The listing builds one solid part. Answer for the finished solid, in the listing's coordinates (mm). Round coordinates to 2 decimals unless told otherwise and drop trailing zeros. Write each loop counter-clockwise with the first axis right and the second up, starting at its lowest first coordinate (ties: lowest second). Pieces come first, ordered by that corner, then holes.
Item 1: Find section B-B on y = 1.8. Give the vertices of the cut face in (x, z).
Item 2: Find section A-A on z = 25. Give the vertices of the cut face in (x, y), then the cut area to 3 significant figures.
Item 3: This flat-tipped pin is pushed along its axis until it touches: pin 1 (3.5 mm diameter, centred on x = 25.83, z = -25.83, fed in from -Y). Where does it stop, or does it pass through?
Item 4: Find the intervals of material crossed by probe 1 along Z at (x, y) = (-25, 3.4); probe 2 along Z at (x, y) = (-28, 2.3); probe 3 along X at (y, z) = (3.1, 28.5), in increasing order.
Autodesk Inventor part; units mm, degrees
ref_plane "YZ Plane" through (0, 0, 0) normal (1, 0, 0) x (0, 1, 0)
ref_plane "XZ Plane" through (0, 0, 0) normal (0, 1, 0) x (-1, 0, 0)
ref_plane "XY Plane" through (0, 0, 0) normal (0, 0, 1) x (1, 0, 0)
sketch "Sketch1" plane through (0, 0, 0) normal (0, 1, 0) x (-1, 0, 0)
  line L0 (25.8285, 25.8285) -> (-25.8285, 25.8285) construction
  line L1 (-25.8285, 25.8285) -> (-25.8285, -25.8285) construction
  line L2 (-25.8285, -25.8285) -> (25.8285, -25.8285) construction
  line L3 (25.8285, -25.8285) -> (25.8285, 25.8285) construction
  line L4 (25.8285, 25.8285) -> (-25.8285, -25.8285) construction
  line L5 (-25.8285, 25.8285) -> (25.8285, -25.8285) construction
  line L6 (31, 26.3139) -> (31, -26.3139)
  line L7 (25.8285, -25.8285) -> (28.6569, -28.6569) construction
  line L8 (28.6569, -28.6569) -> (31, -26.3139)
  line L9 (0, 0) -> (14.4135, 0) construction
  line L10 (25.8285, 25.8285) -> (28.6569, 28.6569) construction
  line L11 (28.6569, 28.6569) -> (31, 26.3139)
  line L12 (-26.3139, 31) -> (26.3139, 31)
  line L13 (28.6569, 28.6569) -> (26.3139, 31)
  line L14 (-28.6569, 28.6569) -> (-26.3139, 31)
  line L15 (-31, -26.3139) -> (-31, 26.3139)
  line L16 (-28.6569, 28.6569) -> (-31, 26.3139)
  line L17 (-28.6569, -28.6569) -> (-31, -26.3139)
  line L18 (26.3139, -31) -> (-26.3139, -31)
  line L19 (-28.6569, -28.6569) -> (-26.3139, -31)
  line L20 (28.6569, -28.6569) -> (26.3139, -31)
  dimension "d0" = 51.657
  dimension "d1" = 51.657
  dimension "d4" = 31
  dimension "d5" = 4
  dimension "d8" = 360
extrude "Extrusion1" add sketch "Sketch1" along normal blind 4
hole "Hole1" at (-25.8285, 0, 25.8285) at (-25.8285, 0, -25.8285) at (25.8285, 0, 25.8285) at (25.8285, 0, -25.8285) direction (0, 1, 0) diameter 4.2 end through all
properties part number "top"
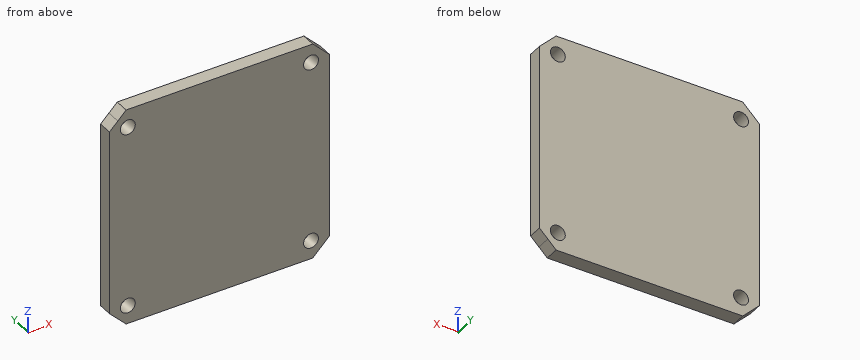
Check values:
1. outline: (-31, -26.31) - (-28.66, -28.66) - (-26.31, -31) - (26.31, -31) - (28.66, -28.66) - (31, -26.31) - (31, 26.31) - (28.66, 28.66) - (26.31, 31) - (-26.31, 31) - (-28.66, 28.66) - (-31, 26.31) - close; hole circle Ø4.2 at (-25.83, -25.83); hole circle Ø4.2 at (-25.83, 25.83); hole circle Ø4.2 at (25.83, -25.83); hole circle Ø4.2 at (25.83, 25.83)
2. outline: (-31, 0) - (-27.76, 0) - (-27.76, 4) - (-31, 4) - close; (-23.9, 0) - (23.9, 0) - (23.9, 4) - (-23.9, 4) - close; (27.76, 0) - (31, 0) - (31, 4) - (27.76, 4) - close
2. area: 217 mm2
3. pin 1: passes through
4. probe 1: z = -31 to -27.76, -23.9 to 23.9, 27.76 to 31
4. probe 2: z = -29.31 to 29.31
4. probe 3: x = -28.81 to 28.81
